Input: dimensioned drawing with shaded views. Units: mm. Origin: part minimum x, y, z. Round coordinates to 2 decimals unless told otherwise and drop trailing zeros. Loops run counter-clockwise (first coordinate to the right, second up) from the corner with the lowest first, then second, coordinate; pieces in that order, holes last. Notation, with made-up numbers: (89.5, 88) - (99.5, 88) arc R10 cw to (99.5, 93) - close; hole circle Ø5 at (84.5, 67.25). An arc over 180 degrees is marked (long way). One line per question, with ' | ' between items.
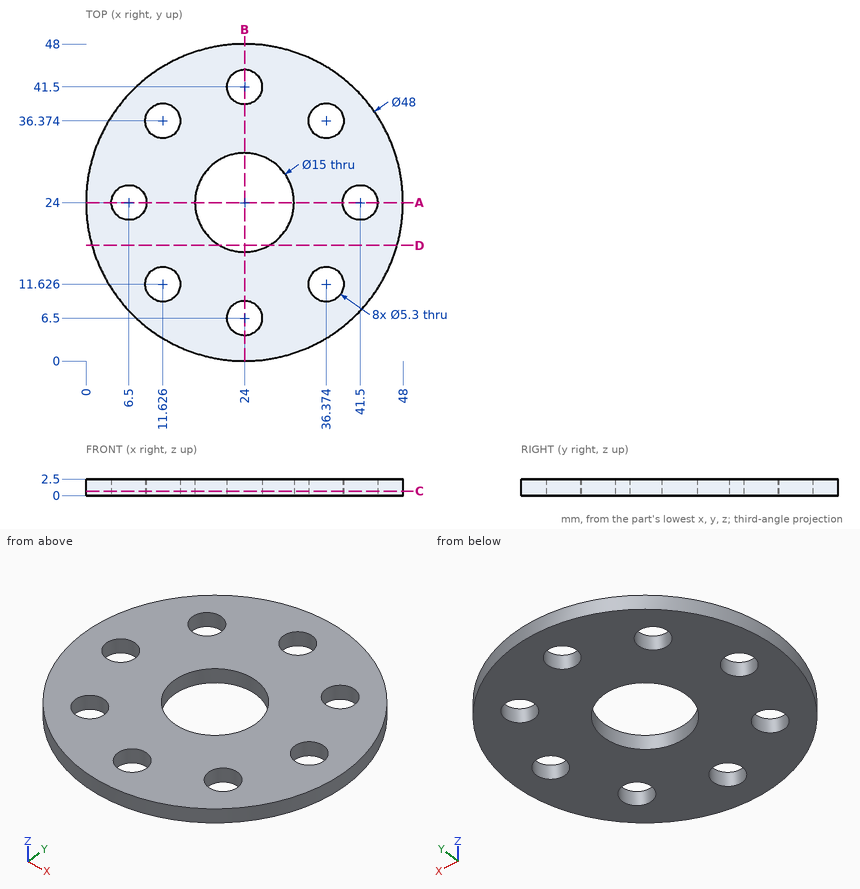
1. Section query C-C, the plane z = 0.65. Give the number of separate pieces and of enclosed holes in the cut face, plus the area to 3 significant figures.
Worked out:
separate pieces: 1 | enclosed holes: 9 | area: 1,460 mm2
2. Material intervals for probe 1 along Y at (x, z) = (24, 1.2); probe 2 along X at (y, z) = (37.5, 2.1) (1 decimal); probe 3 along Y at (x, z) = (7, 1.8), sorted ascending.
Worked out:
probe 1: y = 0 to 3.85, 9.15 to 16.5, 31.5 to 38.85, 44.15 to 48 | probe 2: x = 4.2 to 9.2, 14 to 34, 38.8 to 43.8 | probe 3: y = 7.06 to 21.4, 26.6 to 40.94
3. Section query D-D, the plane y = 17.5. Return loops of the section in (x, z).
Worked out:
outline: (0.9, 0) - (20.26, 0) - (20.26, 2.5) - (0.9, 2.5) - close; (27.74, 0) - (47.1, 0) - (47.1, 2.5) - (27.74, 2.5) - close
4. Contact query for flat-ended pins moving along their axis: P1, Ø1.5, axis at y = 40, z = 1.5, coming from the -X side; P2, Ø5, axis at x = 36.37, y = 11.63, coming from the -Z side. Output: stop coordinate, or through.
Worked out:
P1: stops at x = 5.47 | P2: passes through
5. Section query A-A, the plane y = 24. Return loops of the section in (x, z), plus the area to 3 significant figures.
Worked out:
outline: (0, 0) - (3.85, 0) - (3.85, 2.5) - (0, 2.5) - close; (9.15, 0) - (16.5, 0) - (16.5, 2.5) - (9.15, 2.5) - close; (31.5, 0) - (38.85, 0) - (38.85, 2.5) - (31.5, 2.5) - close; (44.15, 0) - (48, 0) - (48, 2.5) - (44.15, 2.5) - close | area: 56.0 mm2
